Job drawing, mm, ordinate dimensions from the low corner. One solid piece. A direction names the side the tool comes from. Round coordinates to 2 decimals unless told otherwise and drop trailing zeros. Loops run counter-clockwise (first coordinate to the right, second up) from the corner with the lowest first, then second, coordinate; pieces in that order, holes last. Notation, with made-up numbers: M 66.5,-17.75 L 94.5,-17.75 A31 cw 94.5,12.25 Z; hole C 23,-36 d1. An arc over 180 degrees is marked long. Put each result on its own line as item: value. Start each with the question number.
1) Which spindle directions (+Z, -Z, +X, -X, +Y, -Y) get a long thin tool onto all of the face, cutting with end or side? Do the marked faces 1 and 2. Say none if no direction does.
2) Slice it at B-B on z = 8. Give the cut face in (x, y) (1 decimal).
3) Slice it at A-A on x = 127. Give the cut face in (y, z).
4) Drop flat-ended pins along their axis: pin 1 Ø3 at (x, z) = (69.5, 30.5) entering from -Y; pin 2 Ø1 at (y, z) = (93.5, 28.5) entering from -X; pin 3 Ø6 at (x, y) = (75.5, 88) entering from +Z. Give the stop position or say it passes through.
5) Slice it at D-D on x = 181. Give the cut face in (y, z) (1 decimal), then the cut area to 3 significant figures.
6) Probe line 1 along Y through (x, z) = (127, 14); line 2 along Z through (x, y) = (52, 158); line 3 along Z through (x, y) = (67.5, 80). List the from-to ranges inside material, lowest first.
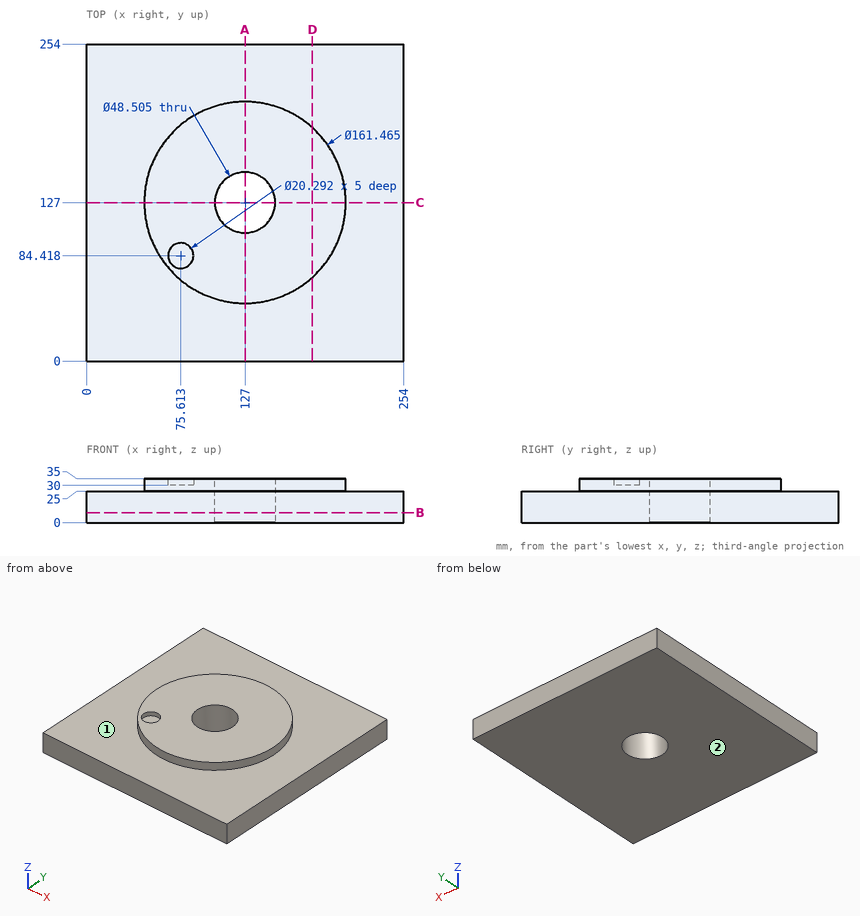
Recorded:
1. face 1: +Z
1. face 2: -Z, +X, -X, +Y, -Y
2. outline: M 0,0 L 254,0 L 254,254 L 0,254 Z; hole C 127,127 d48.5
3. outline: M 0,0 L 102.75,0 L 102.75,35 L 46.27,35 L 46.27,25 L 0,25 Z; M 151.25,0 L 254,0 L 254,25 L 207.73,25 L 207.73,35 L 151.25,35 Z
4. pin 1: stops at y = 68.85
4. pin 2: stops at x = 53.32
4. pin 3: stops at z = 30
5. outline: M 0,0 L 254,0 L 254,25 L 187,25 L 187,35 L 67,35 L 67,25 L 0,25 Z
5. area: 7,550 mm2
6. line 1: y = 0 to 102.75, 151.25 to 254
6. line 2: z = 0 to 25
6. line 3: z = 0 to 30
